Source: CAD feature listing. Evaluate the final solid. Frame: model axes, mm. Round coordinates to 2 decimals unless told otherwise and drop trailing zeros. Loops run counter-clockwise (first coordinate to the right, second up) from the corner with the lowest first, then second, coordinate; pieces in that order, holes last. Notation, with made-up numbers: (15.25, 17) - (53.25, 17) arc R22 cw to (53.25, 33) - close; hole circle Ø9 at (-21.5, -20). An arc over 180 degrees is marked (long way). One line per question, with ' | ' between items. Start each with the question number.
1. Cut plane B-B (z = 6.5). Return loops of the section in (x, y).
2. Cut plane A-A (z = -9). Return loops of the section in (x, y).
3. Mould query, pull axis X, two halves, no side actions, for faces 1 (the flat face through (6.06, -17.08, -3.94)), 2 (the cylindrical face through (26.172, -17.172, -21.895)), 3 (the cylindrical face through (21.046, -8.586, 14.794)). Classes: pulls with the +X half, pulls with the -X half, needs draft (parallel to the pull), parting line crosses it, or undercut.
4. Ray query, line 1 (X direction, y = -33, z = -19); line 2 (Z direction, x = 48, y = -8); line 3 (X direction, y = -7.5, z = -4). Return the intervals inside material, ascending.
5. Pin query (flat end, axial travel): pin 1 (4 mm diameter, centred on x = 11.5, z = 3, fed in from -Y); pin 2 (1 mm diameter, centred on x = 46, z = -11, fed in from -Y); pin 3 (4 mm diameter, centred on x = 13, y = -11, fed in from -Z). Return the tip coordinate at first contact, or that it passes through.
```python
from build123d import *

# Parameters (mm, degrees)
F1_ANGLE = 120


with BuildPart() as f1:
    # F0 (on Front) → F1 (revolve)
    with BuildSketch(Plane.XZ):
        Polygon((25.919337, 20.709641), (15.919337, 20.709641), (15.919337, -14.290359), (35.919337, -14.290359), (35.919337, -29.290359), (55.919337, -29.290359), (55.919337, -11.290359), (35.919337, 8.709641), (25.919337, 8.709641), align=None)
    revolve(axis=Axis((15.919337, 0, 3.209641), (0, 0, -1)), revolution_arc=F1_ANGLE)


solid = f1.part
```
Answers follow:
1) outline: (4.81, -19.23) arc R22.21 ccw to (38.13, 0) - (15.92, 0) - close
2) outline: (-2.94, -32.66) arc R37.71 ccw to (53.63, 0) - (15.92, 0) - close
3) face 1: pulls with the -X half | face 2: undercut | face 3: parting line crosses it
4) line 1: x = -3.13 to 38.52 | line 2: z = -29.29 to -4.35 | line 3: x = 11.59 to 47.76
5) pin 1: stops at y = -27.38 | pin 2: stops at y = -26.82 | pin 3: stops at z = -14.29
